For this review, take the finished solid that the model builds, in its own axes (mm). Coordinates: 2 decimals unless noted, no trailing zeros. Order: outer loops, then holes, each group sorted by start corner. A loop starts at its lowest first (then second) coordinate and runs counter-clockwise, first axis right, second up. Notation, with made-up numbers: (-39.75, 13.5) -> (-29.75, 13.5) arc R28 ccw to (-29.75, 45.5) -> close; hole circle Ø9 at (27.5, 67). An arc over 180 degrees is marked (long way). Return JSON: item names as keys, results as strings. Group by question number.
Item 1: Draft analysis for pull direction Y (two halves, no side actions). For faces 1 (the conical face through (-3.193, 1.854, 3.106)), 2 (the cylindrical face through (0, -2, 2)), 3 (the conical face through (3.193, -1.854, 0.094)), state which applies: +Y half, -Y half, draft (parallel to the pull), parting line (faces both ways), or undercut.
Item 2: For line 1 along Y through (x, z) = (0.75, 1.3); line 2 along Y through (x, z) = (-1.5, 1.9); line 3 along X through (y, z) = (-1.5, 2.5), list the stretches that pass through material, from the lowest coordinate up.
Item 3: Insertion check: pin 1 (1.5 mm diameter, centred on x = 2.5, z = 1.5, fed in from -Y). The pin has a flat end and moves straight along its axis. Give the tip position at first contact, or say it passes through.
Item 4: Take a section at A-A (z = 0.8). Write out the cut boundary in (x, y), then the cut area to 3 significant figures.
```python
from build123d import *

# Parameters (mm, degrees)
SKETCH1_R           = 2
BOSS_EXTRUDE1_DEPTH = 3.2


with BuildPart() as part:
    # Sketch1 → Boss-Extrude1 (new body)
    with BuildSketch(Plane.XY):
        Polygon((0, -4.041451884), (3.5, -2.020725942), (3.5, 2.020725942), (0, 4.041451884), (-3.5, 2.020725942), (-3.5, -2.020725942), align=None)
        Circle(SKETCH1_R, mode=Mode.SUBTRACT)
    extrude(amount=BOSS_EXTRUDE1_DEPTH)

    # Sketch2 → Cut-Revolve1 (revolve, cut)
    with BuildSketch(Plane(origin=(0, 0, 0), x_dir=(0, 0, -1), z_dir=(1, 0, 0)), mode=Mode.PRIVATE) as cut_revolve1_sk:
        Polygon((-3.2, 4.041451884), (-3.2, 3.5), (-2.933333333, 4.041451884), align=None)
        Polygon((-0.266666667, 4.041451884), (0, 4.041451884), (0, 3.5), align=None)
        Polygon((-3.2, 2), (-2.88, 2), (-3.2, 2.32), align=None)
        Polygon((0, 2), (-0.32, 2), (0, 2.32), align=None)
    revolve(cut_revolve1_sk.sketch.rotate(Axis((0, 0, 0), (0, 0, 1)), 90), axis=Axis((0, 0, 0), (0, 0, 1)), mode=Mode.SUBTRACT)


solid = part.part
```
Findings below:
{
 "1": {"face 1": "+Y half", "face 2": "undercut", "face 3": "-Y half"},
 "2": {"line 1": "y = -3.61 to -1.85, 1.85 to 3.61", "line 2": "y = -3.18 to -1.32, 1.32 to 3.18", "line 3": "x = -3.5 to -1.32, 1.32 to 3.5"},
 "3": {"pin 1": "stops at y = -3.03"},
 "4": {"outline": "(-3.5, -2.02) -> (0, -4.04) -> (3.5, -2.02) -> (3.5, 2.02) -> (0, 4.04) -> (-3.5, 2.02) -> close; hole circle Ø4 at (0, 0)", "area": "29.9 mm2"}
}
